Check sheet for the drawn part. Datum: minimum x, y, z corner. Units: mm. A direction names the side the tool comes from. Round coordinates to 2 decimals unless told otherwise and drop trailing zeros. Order: outer loops, then holes, each group sorted by start corner. A loop starts at its lowest first (then second) coordinate and runs counter-clockwise, first axis right, second up. Notation, with made-up numbers: (-3.75, 1) - (49.25, 1) arc R22 cw to (49.25, 39) - close; hole circle Ø8 at (-33, 78). An arc over 180 degrees is marked (long way). Write each question's results on one line, items separated by ' | '.
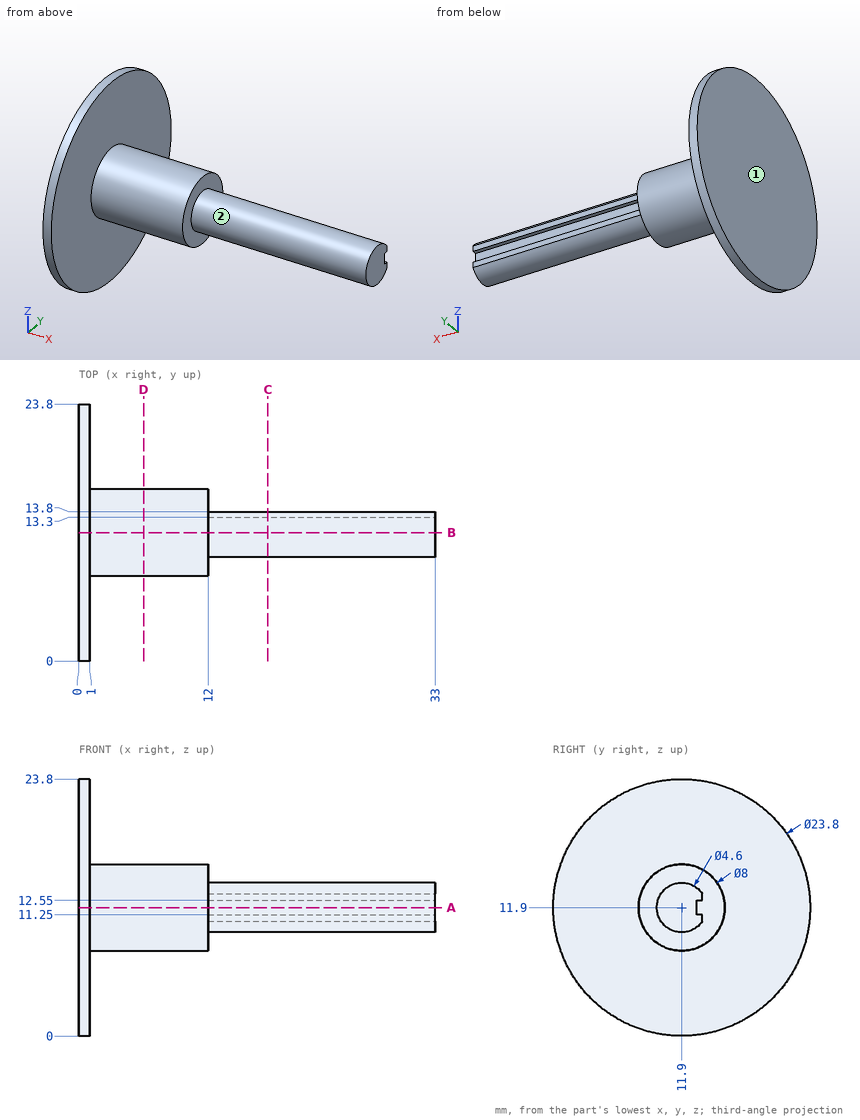
(1) Section check C-C (x = 17.5). Record the cut outline in (y, z), then the cut area to 3 significant figures.
Answers follow:
outline: (13.3, 11.25) - (13.3, 12.55) - (13.8, 12.55) - (13.8, 13.2) arc R2.3 ccw (long way) to (13.8, 10.6) - (13.8, 11.25) - close | area: 15.3 mm²
(2) Access from +Z, -Z, +X, -X, +Y, -Y to the whole of each face (thin tool, end or side, straight path). Record for the marked faces 1 and 2.
Answers follow:
face 1: +Z, -Z, -X, +Y, -Y | face 2: +X
(3) Depth check by flat-ended pin: pin 1 Ø2 at (x, y) = (6, 13) entering from +Z; pin 2 Ø6 at (x, z) = (14, 13.5) entering from -Y; pin 3 Ø12 at (x, z) = (8.5, 5.5) entering from +Y. Enter the tip coordinate at first touch or a pass-through.
Answers follow:
pin 1: z = 15.9 | pin 2: y = 7.9 | pin 3: y = 15.88
(4) Material ranges on line 1 (X direction, y = 1, z = 10); line 2 (X direction, y = 12, z = 15.75); line 3 (Z direction, x = 26, y = 10), recorded low to high.
Answers follow:
line 1: 0 to 1 | line 2: 0 to 12 | line 3: 10.6 to 13.2
(5) Section check D-D (x = 6). Record the cut outline in (y, z), then the cut area to 3 significant figures.
Answers follow:
outline: circle Ø8 at (11.9, 11.9) | area: 50.3 mm²
(6) Section check B-B (y = 11.9). Record the cut outline in (x, z), then the cut area to 3 significant figures.
Answers follow:
outline: (0, 0) - (1, 0) - (1, 7.9) - (12, 7.9) - (12, 9.6) - (33, 9.6) - (33, 14.2) - (12, 14.2) - (12, 15.9) - (1, 15.9) - (1, 23.8) - (0, 23.8) - close | area: 208 mm²
(7) Section check A-A (z = 11.9). Record the cut outline in (x, y), then the cut area to 4 significant figures.
Answers follow:
outline: (0, 0) - (1, 0) - (1, 7.9) - (12, 7.9) - (12, 9.6) - (33, 9.6) - (33, 13.3) - (12, 13.3) - (12, 15.9) - (1, 15.9) - (1, 23.8) - (0, 23.8) - close | area: 189.5 mm²
